```python
from build123d import *

# Parameters (mm, degrees)
F0_W      = 118
F0_H      = 75
F1_DEPTH  = 2
F2_W      = 48
F2_H      = 28
F2_R      = 2.5
F3_DEPTH  = 25
F4_W      = 2
F4_H      = 75
F5_DEPTH  = 47
F6_R      = 2
F7_R      = 2.5
F8_DEPTH  = 25
F9_R      = 2.5
F10_DEPTH = 25


with BuildPart() as f1:
    # F0 (on Top) → F1 (new body)
    with BuildSketch(Plane.XY):
        Rectangle(F0_W, F0_H)
    extrude(amount=F1_DEPTH)

    # F2 (on face) → F3 (cut)
    with BuildSketch(Plane.XY.offset(2)):
        with Locations((10, -11.5)):
            Rectangle(F2_W, F2_H)
        with Locations((10, -31.5)):
            Circle(F2_R)
        with Locations((10, 8.5)):
            Circle(F2_R)
    extrude(amount=-F3_DEPTH, mode=Mode.SUBTRACT)

    # F4 (on face) → F5 (join)
    with BuildSketch(Plane(origin=(0, 0, 0), x_dir=(1, 0, 0), z_dir=(0, 0, -1))):
        with Locations((-58, 0)):
            Rectangle(F4_W, F4_H)
        with Locations((58, 0)):
            Rectangle(F4_W, F4_H)
    extrude(amount=F5_DEPTH)

    # F6
    f6_edges = [f1.edges().sort_by_distance(p)[0] for p in [
        (59, 0, 2),
        (-59, 0, 2),
    ]]
    fillet(f6_edges, radius=F6_R)

    # F7 (on face) → F8 (cut)
    with BuildSketch(Plane(origin=(-59, 0, 0), x_dir=(0, -1, 0), z_dir=(-1, 0, 0))):
        with Locations((-25.5, -37)):
            Circle(F7_R)
    extrude(amount=-F8_DEPTH, mode=Mode.SUBTRACT)

    # F9 (on face) → F10 (cut)
    with BuildSketch(Plane.YZ.offset(59)):
        with Locations((25.5, -37)):
            Circle(F9_R)
    extrude(amount=-F10_DEPTH, mode=Mode.SUBTRACT)


solid = f1.part
```
Source: CAD feature listing. Evaluate the final solid. Frame: model axes, mm. A direction names the side the tool comes from. Round coordinates to 2 decimals unless told otherwise and drop trailing zeros. Write each loop counter-clockwise with the first axis right and the second up, starting at its lowest first coordinate (ties: lowest second). Pieces come first, ordered by that corner, then holes. Notation, with made-up numbers: M 8,66.25 L 66,66.25 A15 ccw 66,85.25 Z; hole C -24,-4.75 d1. An arc over 180 degrees is marked long. Answer as a JSON object with one key per item and string values. Group by question number.
(1) Ray query, line 1 (X direction, y = 24, z = -2); line 2 (Y direction, x = 10, z = 1); line 3 (Z direction, x = -19, y = 26). Return the intervals inside material, ascending. Write a range as [from, to].
(2) Section query B-B on y = -19.5. Output: boundary loops of the cut face in (x, z), then the cut area to 3 significant figures.
(3) Reachability of faces 5 (the flat face through (-57, 1, -23)), 6 (the cylindrical face through (10, -29, 1)) from +Z, -Z, +X, -X, +Y, -Y: full face, straight path, thin tool, end or side. Return the list, or none.
(4) Section query C-C on z = -22. Output: boundary loops of the cut face in (x, y).
(5) Mould query, pull axis Y, two halves, no side actions, for faces 1 (the flat face through (-26, 37.5, 1)), 2 (the cylindrical face through (-58, 27, -35)), 3 (the cylindrical face through (9.46, 6.06, 1.01)), 4 (the flat face through (-26, -37.5, 1)). Classes: +Y half, -Y half, draft (parallel to the pull), parting line (faces both ways), or undercut.
(6) Section query A-A on y = 25.5. Output: boundary loops of the cut face in (x, z).
(7) Section query D-D on x = 1. Output: boundary loops of the cut face in (y, z), then the cut area to 3 significant figures.
(8) First-contact query: pin 1 (3 mm diameter, centred on y = 25.5, z = -37, fed in from -X); pin 2 (12 mm diameter, centred on x = -0.5, y = 7.5, fed in from -Z); pin 3 (1.6 mm diameter, centred on y = -15, z = 1.5, fed in from +X). Flat tips, straight axial feed; report the tip coordinate or a pass-through.
Computed values:
{
 "1": {"line 1": "[-59, -57], [57, 59]", "line 2": "[-37.5, -34], [-29, -25.5], [2.5, 6], [11, 37.5]", "line 3": "[0, 2]"},
 "2": {"outline": "M -59,-47 L -57,-47 L -57,0 L -14,0 L -14,2 L -57,2 A2 ccw -59,0 Z; M 34,0 L 57,0 L 57,-47 L 59,-47 L 59,0 A2 ccw 57,2 L 34,2 Z", "area": "326 mm^2"},
 "3": {"face 5": "-Z, +Y, -Y", "face 6": "+Z, -Z"},
 "4": {"outline": "M -59,-37.5 L -57,-37.5 L -57,37.5 L -59,37.5 Z; M 57,-37.5 L 59,-37.5 L 59,37.5 L 57,37.5 Z"},
 "5": {"face 1": "+Y half", "face 2": "undercut", "face 3": "undercut", "face 4": "-Y half"},
 "6": {"outline": "M -59,-47 L -57,-47 L -57,-39.5 L -59,-39.5 Z; M -59,-34.5 L -57,-34.5 L -57,0 L 57,0 L 57,-34.5 L 59,-34.5 L 59,0 A2 ccw 57,2 L -57,2 A2 ccw -59,0 Z; M 57,-47 L 59,-47 L 59,-39.5 L 57,-39.5 Z"},
 "7": {"outline": "M -37.5,0 L -25.5,0 L -25.5,2 L -37.5,2 Z; M 2.5,0 L 37.5,0 L 37.5,2 L 2.5,2 Z", "area": "94.0 mm^2"},
 "8": {"pin 1": "through", "pin 2": "z = 0", "pin 3": "x = 58.87"}
}
